Here's the drawing with two shaded views (mm, measured from the low corner). I have some questions. Round coordinates to 2 decimals unless told otherwise and drop trailing zeros. Order: outer loops, then holes, each group sorted by start corner. A loop starts at its lowest first (then second) coordinate and runs counter-clockwise, first axis right, second up. Notation, with made-up numbers: (28.5, 31.5) - (42.5, 31.5) arc R25 cw to (42.5, 70.5) - close; hole circle Ø9 at (53, -39.75). An arc over 180 degrees is marked (long way). One line per item, written item: value.
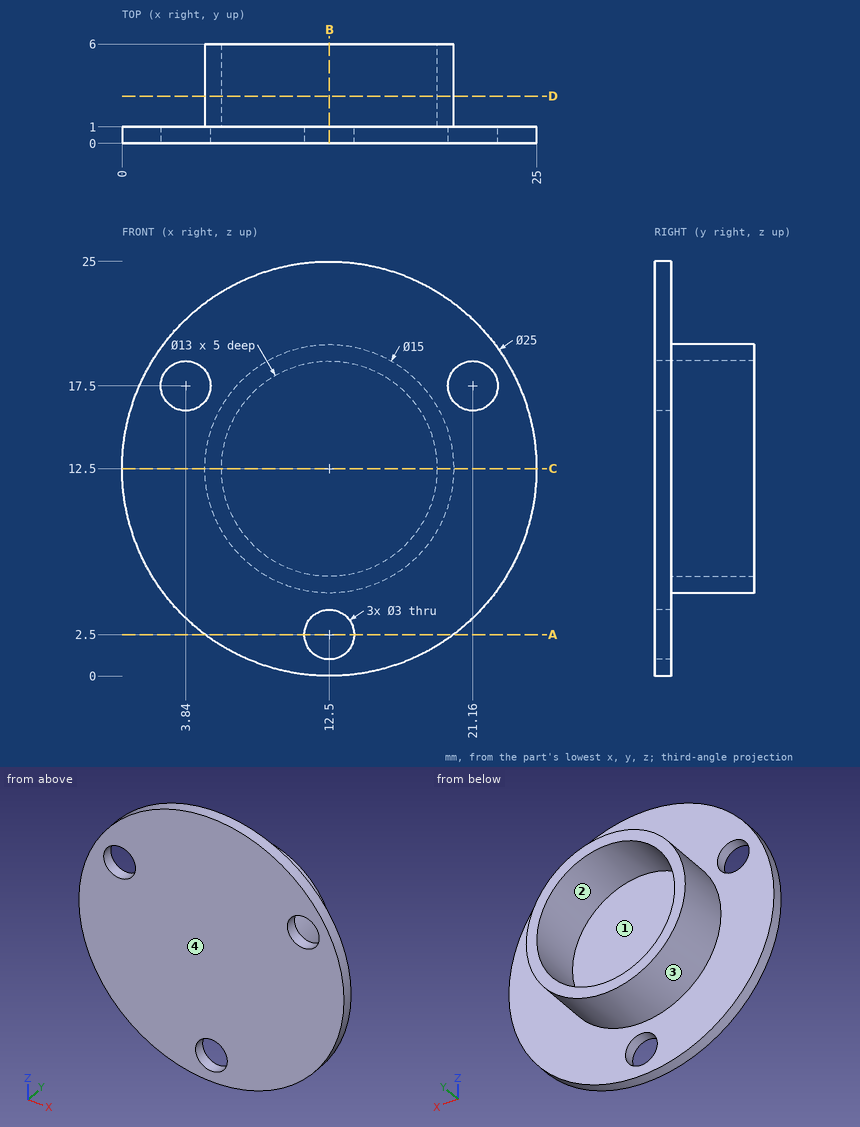
Q1. We'd pull the mould along Z, two halves only. Please class the marked faces 1, 2, 3 and 4: released by +Z, released by -Z, zero draft, split by the parting line, or undercut.
Results list:
face 1: undercut
face 2: undercut
face 3: split by the parting line
face 4: zero draft
Q2. If we section it at C-C, the plane z = 12.5: Please give me the cut outline in (x, y), then the cut area to 3 significant figures.
Results list:
outline: (0, 0) - (25, 0) - (25, 1) - (20, 1) - (20, 6) - (19, 6) - (19, 1) - (6, 1) - (6, 6) - (5, 6) - (5, 1) - (0, 1) - close
area: 35.0 mm²
Q3. If we section it at D-D, the plane y = 2.85: Please give me the cut outline in (x, z).
Results list:
outline: circle Ø15 at (12.5, 12.5); hole circle Ø13 at (12.5, 12.5)
Q4. If I drill on line 1 along X through (y, z) = (5.1, 12.25) (1 decimal); line 2 along X through (y, z) = (0.2, 2.5); line 3 along X through (y, z) = (0.3, 17.5), over which ranges is the centre line in solid material (lowest first)?
Results list:
line 1: 5 to 6, 19 to 20
line 2: 5 to 11, 14 to 20
line 3: 1.04 to 2.34, 5.34 to 19.66, 22.66 to 23.96
Q5. If we section it at A-A, the plane z = 2.5: Please give me the cut outline in (x, y).
Results list:
outline: (5, 0) - (11, 0) - (11, 1) - (5, 1) - close; (14, 0) - (20, 0) - (20, 1) - (14, 1) - close
Q6. Will this pin go through, and if not, where does the flat tip stop? pin 1 (3 mm diameter, centred on x = 8, z = 22, fed in from +Y).
Results list:
pin 1: y = 1
Q7. If we section it at B-B, the plane x = 12.5: Please give me the cut outline in (y, z).
Results list:
outline: (0, 0) - (1, 0) - (1, 1) - (0, 1) - close; (0, 4) - (1, 4) - (1, 5) - (6, 5) - (6, 6) - (1, 6) - (1, 19) - (6, 19) - (6, 20) - (1, 20) - (1, 25) - (0, 25) - close
